Check sheet for the modelled part. Datum: model origin and axes. Units: mm. A direction names the side the tool comes from. Give positions to 0.01 mm unless a question says otherwise; leave off trailing zeros. Loops run counter-clockwise (first coordinate to the right, second up) from the corner with the lowest first, then second, coordinate; pieces in that order, holes last. Notation, with made-up numbers: (-20, -22.5) - (26, -22.5) arc R32 ccw to (26, 6.5) - close; hole circle Ø6 at (-34.75, 34). An arc over 180 degrees is marked (long way). Use CSV: the item, a comma, the result in double quotes.
from build123d import *

# Parameters (mm, degrees)
BOSS_EXTRUDE1_DEPTH = 2
CUT_EXTRUDE1_REACH  = 20.035
SKETCH2_R           = 1.5
SKETCH3_W           = 2
SKETCH3_H           = 5
BOSS_EXTRUDE2_DEPTH = 14.3
BOSS_EXTRUDE3_DEPTH = 2
CUT_EXTRUDE2_REACH  = 27.615
SKETCH5_R           = 1.1
CHAMFER1_SIZE       = 1


with BuildPart() as part:
    # Sketch1 → Boss-Extrude1 (new body)
    with BuildSketch(Plane(origin=(0, 0, 0), x_dir=(1, 0, 0), z_dir=(0, 1, 0))):
        Polygon((-6, -16.5), (6, -16.5), (7, -16.5), (7, 16.5), (6, 16.5), (-6, 16.5), (-6, 11.5), (6, 11.5), (6, -11.5), (-6, -11.5), align=None)
    extrude(amount=BOSS_EXTRUDE1_DEPTH)

    # Sketch2 → Cut-Extrude1 (cut, up to next)
    with BuildSketch(Plane(origin=(0, 2, 0), x_dir=(1, 0, 0), z_dir=(0, 1, 0)), mode=Mode.PRIVATE) as cut_extrude1_sk1:
        with Locations(Location((0, -14, 0), (0, 0, 270))):
            Circle(SKETCH2_R)
    cut_extrude1_tool1 = extrude(cut_extrude1_sk1.sketch, amount=-CUT_EXTRUDE1_REACH, mode=Mode.PRIVATE) & part.part
    # Sketch2 → Cut-Extrude1 (cut, up to next)
    with BuildSketch(Plane(origin=(0, 2, 0), x_dir=(1, 0, 0), z_dir=(0, 1, 0)), mode=Mode.PRIVATE) as cut_extrude1_sk2:
        with Locations(Location((0, 14, 0), (0, 0, 270))):
            Circle(SKETCH2_R)
    cut_extrude1_tool2 = extrude(cut_extrude1_sk2.sketch, amount=-CUT_EXTRUDE1_REACH, mode=Mode.PRIVATE) & part.part
    add(cut_extrude1_tool1.solids().sort_by_distance((0, 2, 14))[0], mode=Mode.SUBTRACT)
    add(cut_extrude1_tool2.solids().sort_by_distance((0, 2, -14))[0], mode=Mode.SUBTRACT)

    # Sketch3 → Boss-Extrude2 (add)
    with BuildSketch(Plane(origin=(0, 2, 0), x_dir=(1, 0, 0), z_dir=(0, 1, 0))):
        with Locations((-5, 14)):
            Rectangle(SKETCH3_W, SKETCH3_H)
        Polygon((7, 16.5), (5, 16.5), (5, 11.5), (6, 11.5), (6, -11.5), (5, -11.5), (5, -16.5), (7, -16.5), (7, -11.5), (7, 11.5), align=None)
        with Locations((-5, -14)):
            Rectangle(SKETCH3_W, SKETCH3_H)
    extrude(amount=BOSS_EXTRUDE2_DEPTH)

    # Sketch4 → Boss-Extrude3 (add)
    with BuildSketch(Plane(origin=(0, 16.3, 0), x_dir=(1, 0, 0), z_dir=(0, 1, 0))):
        Polygon((6, 11.5), (6, -11.5), (-6, -11.5), (-6, -16.5), (7, -16.5), (7, 16.5), (-6, 16.5), (-6, 11.5), align=None)
    extrude(amount=BOSS_EXTRUDE3_DEPTH)

    # Sketch5 → Cut-Extrude2 (cut, up to next)
    with BuildSketch(Plane(origin=(0, 18.3, 0), x_dir=(1, 0, 0), z_dir=(0, 1, 0)), mode=Mode.PRIVATE) as cut_extrude2_sk1:
        with Locations(Location((0, 14, 0), (0, 0, 270))):
            Circle(SKETCH5_R)
    cut_extrude2_tool1 = extrude(cut_extrude2_sk1.sketch, amount=-CUT_EXTRUDE2_REACH, mode=Mode.PRIVATE) & part.part
    # Sketch5 → Cut-Extrude2 (cut, up to next)
    with BuildSketch(Plane(origin=(0, 18.3, 0), x_dir=(1, 0, 0), z_dir=(0, 1, 0)), mode=Mode.PRIVATE) as cut_extrude2_sk2:
        with Locations(Location((0, -14, 0), (0, 0, 270))):
            Circle(SKETCH5_R)
    cut_extrude2_tool2 = extrude(cut_extrude2_sk2.sketch, amount=-CUT_EXTRUDE2_REACH, mode=Mode.PRIVATE) & part.part
    add(cut_extrude2_tool1.solids().sort_by_distance((0, 18.3, -14))[0], mode=Mode.SUBTRACT)
    add(cut_extrude2_tool2.solids().sort_by_distance((0, 18.3, 14))[0], mode=Mode.SUBTRACT)

    # Chamfer1
    chamfer1_edges = [part.edges().sort_by_distance(p)[0] for p in [
        (-6, 9.15, -11.5),
        (-6, 9.15, -16.5),
        (7, 9.15, -16.5),
        (7, 9.15, 16.5),
        (-6, 9.15, 16.5),
        (-6, 9.15, 11.5),
    ]]
    chamfer(chamfer1_edges, length=CHAMFER1_SIZE)


solid = part.part
1. Sectioned sample at D-D, the plane x = -3.5. Record the boundary of the cut face in (y, z), and give its area (3 significant figures).
Completed:
outline,"(0, -16.5) - (2, -16.5) - (2, -11.5) - (0, -11.5) - close; (0, 11.5) - (2, 11.5) - (2, 16.5) - (0, 16.5) - close; (16.3, -16.5) - (18.3, -16.5) - (18.3, -11.5) - (16.3, -11.5) - close; (16.3, 11.5) - (18.3, 11.5) - (18.3, 16.5) - (16.3, 16.5) - close"
area,"40.0 mm²"
2. Set-up check for faces 1 (the face through (6, 9, 0)), 2 (the face through (1.4, 16.3, -14)), 3 (the face through (5.5, 9, -16.5)): record each of +Z, -Z, +X, -X, +Y, -Y from which the full face is reachable in a straight line by a thin tool's end or side.
Completed:
face 1,"-X, +Y, -Y"
face 2,"+Z, -Z"
face 3,"-Z, +X, -X, +Y, -Y"
3. Scan lines: line 1 along X through (y, z) = (1.05, -14); line 2 along Y through (x, z) = (1.75, -14); line 3 along X through (y, z) = (7, 13.5). Record each from-to range of solid material in increasing order.
Completed:
line 1,"x = -6 to -1.5, 1.5 to 7"
line 2,"y = 0 to 2, 16.3 to 18.3"
line 3,"x = -6 to -4, 5 to 7"
4. Sectioned sample at A-A, the plane z = 14. Record the boundary of the cut face in (x, y).
Completed:
outline,"(-6, 0) - (-1.5, 0) - (-1.5, 2) - (-4, 2) - (-4, 16.3) - (-1.1, 16.3) - (-1.1, 18.3) - (-6, 18.3) - close; (1.1, 16.3) - (5, 16.3) - (5, 2) - (1.5, 2) - (1.5, 0) - (7, 0) - (7, 18.3) - (1.1, 18.3) - close"
5. Release check for a two-part mould opening along X. For faces 4 (the face through (6.5, 9, 16)), 5 (the face through (-4.5, 9, -11.5)), 6 (the face through (-5.5, 9.3, -12)), 7 (the face through (0.07, 1.01, 12.5)) record: released by +X, released by -X, zero draft, split by the parting line, or undercut.
Completed:
face 4,"released by +X"
face 5,"zero draft"
face 6,"released by -X"
face 7,"undercut"
6. Go/stop test with a flat-tipped pin: pin 1 Ø5 at (y, z) = (6.5, 2) entering from -X. Record where the tip stops, or that it passes through.
Completed:
pin 1,"stops at x = 6"
7. Sectioned sample at B-B, the plane x = 0. State how many separate pieces and enclosed holes the cut face has, and give its area (3 significant figures).
Completed:
separate pieces,"8"
enclosed holes,"0"
area,"19.2 mm²"
8. Sectioned sample at C-C, the plane y = 11.5. Record the boundary of the cut face in (x, z), and give its area (3 significant figures).
Completed:
outline,"(-6, -15.5) - (-5, -16.5) - (-4, -16.5) - (-4, -11.5) - (-5, -11.5) - (-6, -12.5) - close; (-6, 12.5) - (-5, 11.5) - (-4, 11.5) - (-4, 16.5) - (-5, 16.5) - (-6, 15.5) - close; (5, -16.5) - (6, -16.5) - (7, -15.5) - (7, 15.5) - (6, 16.5) - (5, 16.5) - (5, 11.5) - (6, 11.5) - (6, -11.5) - (5, -11.5) - close"
area,"60.0 mm²"
